Model file for the job. Use its own axes, mm. Face numbers are marked on the shaded views. A direction names the side the tool comes from. Give positions to 0.01 mm unless a question says otherwise; leave off trailing zeros. Order: outer loops, then holes, each group sorted by start corner. A loop starts at its lowest first (then second) coordinate and runs counter-clockwise, first axis right, second up. Notation, with made-up numbers: M 22.5,10.5 L 76.5,10.5 A10 ccw 76.5,14.5 Z; hole C 79,4.25 d1. An arc over 180 degrees is marked long. Return JSON: item names as keys, results as strings. Group by question number.
1. Wall check: probe 1 along Y at (x, z) = (-43.5, -28); probe 2 along X at (y, z) = (0, 12); probe 3 along Y at (x, z) = (0, 0). Give the ranges that are in metal, low to high. Write a range as [from, to].
2. Slice it at D-D on z = -33. List the corners of the cut face in (x, y), then the cut area to 3 significant figures.
3. Slice it at A-A on x = -67. List the corners of the cut face in (y, z).
4. Slice it at B-B on y = 102. List the corners of the cut face in (x, z), then the cut area to 3 significant figures.
5. Pin check, flat tips, straight feed: pin 1 (1 mm diameter, centred on x = -23, z = 48, fed in from -Y); pin 2 (6 mm diameter, centred on y = 93.5, z = 31, fed in from -X); pin 3 (16 mm diameter, centred on y = 103.5, z = -31, fed in from -X). Stop position of each tip, or through.
6. 3-axis set-ups, long thin cutter, end or side, ignore diameter. For the marked faces 5, 6 and 7: which of +Z, -Z, +X, -X, +Y, -Y reach the whole face in a straight line?
7. Two-plate mould, pull along Y, no slides. Class the marked faces 1, 2, 3 and 4: released by +Y, released by -Y, zero draft, split by the parting line, or undercut.
8. Slice it at C-C on z = 51. List the corners of the cut face in (x, y), then the cut area to 3 significant figures.
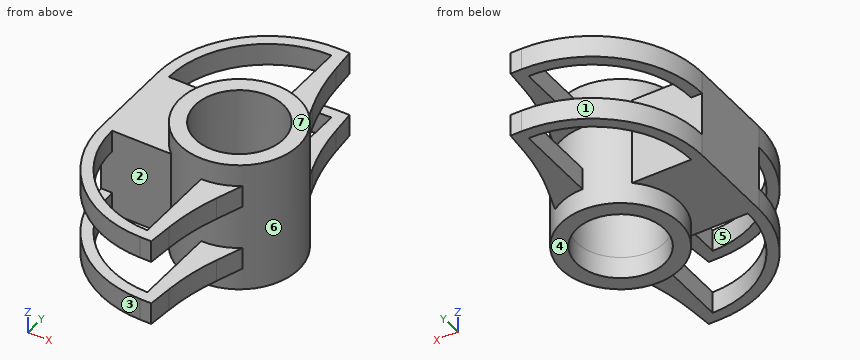
Autodesk Inventor part; units mm, degrees
ref_plane "YZ Plane" through (0, 0, 0) normal (1, 0, 0) x (0, 1, 0)
ref_plane "XZ Plane" through (0, 0, 0) normal (0, 1, 0) x (-1, 0, 0)
sketch "Sketch1" plane through (0, 0, 0) normal (0, 0, 1) x (1, 0, 0)
  circle A0 centre (0, 0) radius 20
  circle A1 centre (0, 0) radius 27
  line L0 (-27, 0) -> (-50, 0) construction
  line L1 (-50, 20) -> (-50, -20)
  line L2 (-50, 20) -> (-18.1384, 20)
  line L3 (-50, -20) -> (-18.1384, -20)
  dimension "d0" = 40
  dimension "d1" = 54
  dimension "d2" = 23
  dimension "d3" = 50
  dimension "d4" = 40
  dimension "d5" = 20
  dimension "d6" = 20
sketch "Sketch2" plane through (0, 0, 0) normal (0, 0, 1) x (1, 0, 0)
  point P0 (0, 0)
sketch "Sketch3" plane through (0, 0, 0) normal (0, 0, 1) x (1, 0, 0)
  point P0 (0, 0)
extrude "Extrusion1" add sketch "Sketch1" along normal mid plane 40
sketch "Sketch4" plane through (0, 0, 20) normal (0, 0, 1) x (1, 0, 0)
  circle A0 centre (0, 0) radius 20
  circle A1 centre (0, 0) radius 27
  dimension "d9" = 40
  dimension "d10" = 54
extrude "Extrusion2" add sketch "Sketch4" along normal blind 10
sketch "Sketch5" plane through (0, 0, -20) normal (0, 0, -1) x (-1, 0, 0)
  circle A0 centre (0, 0) radius 20
  circle A1 centre (0, 0) radius 27
  dimension "d13" = 40
  dimension "d14" = 54
extrude "Extrusion3" add sketch "Sketch5" along normal blind 10
sketch "Sketch6" plane through (0, 0, 0) normal (0, 0, 1) x (1, 0, 0)
  point P0 (0, 0)
ref_plane "Work Plane1" through (0, 0, 10) normal (0, 0, 1) x (1, 0, 0)
sketch "Sketch7" plane through (0, 0, 10) normal (0, 0, 1) x (1, 0, 0)
  circle A0 centre (0, 0) radius 20
  line L0 (-50, 20) -> (-18.1384, 20)
  arc A1 (0, 70) -> (-50, 20) centre (0, 20) ccw
  arc A2 (0, 65) -> (-45, 20) centre (0, 20) ccw
  line L1 (0, 65) -> (0, 27)
  circle A3 centre (0, 0) radius 27
  line L2 (0, 70) -> (5, 70)
  line L3 (5, 70) -> (5.9668, 58.8209)
  line L4 (11.398, 33.8671) -> (15.6186, 22.0241)
  arc A4 (5.9668, 58.8209) -> (11.398, 33.8671) centre (105.5949, 67.4369) ccw
  point P0 (7.7299, 38.4334)
  point P1 (5, 51.8198)
  dimension "d18" = 50
  dimension "d19" = 45
  dimension "d20" = 38
  dimension "d21" = 5
  dimension "d22" = 5
  dimension "d23" = 31.5666
  dimension "d24" = 94.943
  dimension "d25" = 29.7957
  dimension "d26" = 165.328
  dimension "d27" = 22.1057
  dimension "d28" = 100
extrude "Extrusion4" add sketch "Sketch7" along normal blind 10 contours A1 L2 L3 A4 L4 A3 L1 A2 L0
mirror "Mirror1" about plane through (0, 0, 0) normal (0, 0, 1) of "Extrusion4"
mirror "Mirror2" about plane through (0, 0, 0) normal (0, 1, 0) of "Extrusion4", "Mirror1"
scale "Scale1" factors (2, 2, 2) then translate (0, 0, 0) bodies 1
properties part number "project part" material "Aluminum 6061"
Result:
{
 "1": {"probe 1": "y = [-130.04, -118.79], [-40, 40], [118.79, 130.04]", "probe 2": "x = [-100, -40], [40, 54]", "probe 3": "y = [-54, -40], [40, 54]"},
 "2": {"outline": "M -100,-40 A100 ccw 0,-140 L 10,-140 L 11.93,-117.64 A200 cw 22.8,-67.73 L 31.24,-44.05 A54 ccw 31.24,44.05 L 22.8,67.73 A200 cw 11.93,117.64 L 10,140 L 0,140 A100 ccw -100,40 Z; hole M -90,-40 A90 ccw 0,-130 L 0,-54 A54 cw -36.28,-40 Z; hole M -90,40 L -36.28,40 A54 cw 0,54 L 0,130 A90 ccw Z; hole C 0,0 d80", "area": "14,200 mm2"},
 "3": {"outline": "M -114.24,-40 L -100.09,-40 L -100.09,-20 L -114.24,-20 Z; M -114.24,20 L -100.09,20 L -100.09,40 L -114.24,40 Z; M -40,-40 L 40,-40 L 40,40 L -40,40 Z; M 100.09,-40 L 114.24,-40 L 114.24,-20 L 100.09,-20 Z; M 100.09,20 L 114.24,20 L 114.24,40 L 100.09,40 Z"},
 "4": {"outline": "M -78.46,-40 L -65.24,-40 L -65.24,-20 L -78.46,-20 Z; M -78.46,20 L -65.24,20 L -65.24,40 L -78.46,40 Z; M 0,-40 L 13.91,-40 L 13.91,-20 L 0,-20 Z; M 0,20 L 13.91,20 L 13.91,40 L 0,40 Z", "area": "1,090 mm2"},
 "5": {"pin 1": "stops at y = -49.09", "pin 2": "stops at x = -86.31", "pin 3": "stops at x = -83.19"},
 "6": {"face 5": "+Z, -Z", "face 6": "none", "face 7": "+Z, +X, -X, +Y, -Y"},
 "7": {"face 1": "released by +Y", "face 2": "undercut", "face 3": "released by -Y", "face 4": "zero draft"},
 "8": {"outline": "C 0,0 d108; hole C 0,0 d80", "area": "4,130 mm2"}
}
